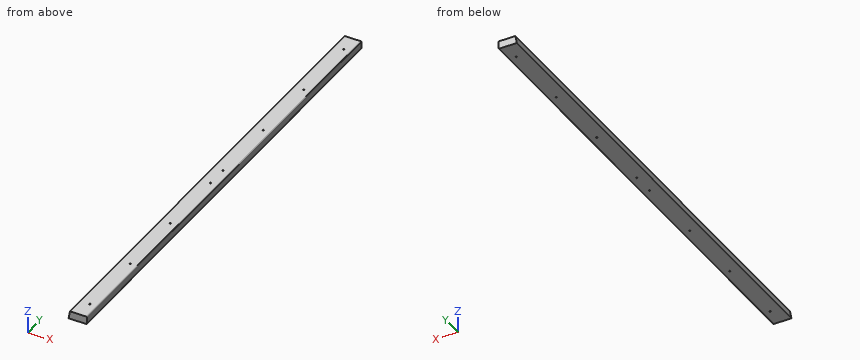
```python
from build123d import *

# Parameters (mm, degrees)
BOSS_EXTRUDE1_DEPTH         = 2362.2
F_1_4_0_25_DIAMETER_HOLE1_D = 6.35
FILLET2_R                   = 3.175


with BuildPart() as part:
    # Sketch1 → Boss-Extrude1 (new body)
    with BuildSketch(Plane(origin=(0, 0, 0), x_dir=(1, 0, 0), z_dir=(0, 1, 0))):
        Polygon((-44.45, 19.05), (-37.731942035, -19.05), (44.45, -19.05), (44.45, 19.05), align=None)
    extrude(amount=BOSS_EXTRUDE1_DEPTH)

    # 1/4 (0.25) Diameter Hole1 (through all)
    with Locations(Plane(origin=(0, 0, 19.05), x_dir=(-1, 0, 0), z_dir=(0, 0, 1))):
        with Locations((-8.817444165, -88.9), (-8.817444165, -434.975), (-8.817444165, -781.05), (-8.817444165, -1127.125)):
            f_1_4_0_25_diameter_hole1 = Hole(F_1_4_0_25_DIAMETER_HOLE1_D / 2)

    # Fillet2
    fillet2_edges = [part.edges().sort_by_distance(p)[0] for p in [
        (44.45, 1181.1, 19.05),
        (44.45, 1181.1, -19.05),
    ]]
    fillet(fillet2_edges, radius=FILLET2_R)

    # Mirror1: 1/4 (0.25) Diameter Hole1 across plane
    add(f_1_4_0_25_diameter_hole1.mirror(Plane(origin=(0, 1181.1, 0), x_dir=(0, 0, 1), z_dir=(0, -1, 0))), mode=Mode.SUBTRACT)


solid = part.part
```
Part model, mm, in its own coordinate system. Coordinates: 2 decimals unless noted, no trailing zeros. Order: outer loops, then holes, each group sorted by start corner. A loop starts at its lowest first (then second) coordinate and runs counter-clockwise, first axis right, second up. Notation, with made-up numbers: (10, 20.25) - (61, 20.25) arc R17 cw to (61, 32.25) - close; hole circle Ø8 at (64, 88.5). An arc over 180 degrees is marked (long way). Return JSON: item names as keys, results as strings. Group by question number.
Item 1: Cut at A-A (y = 1508). List the corners of the cut face in (x, z) (3 decimals), plus the area to 3 significant figures.
Item 2: Cut at B-B (z = 1). State how many separate pieces and enclosed holes the cut face has, plus the area to 3 significant figures.
Item 3: Drill centre lines: probe 1 along X at (y, z) = (1581, 10); probe 2 along X at (y, z) = (88.9, 1); probe 3 along X at (y, z) = (196, -17). Where is each one in solid material? Low to high. Write a range as from..to.
Item 4: Pin check, flat tip, straight feed: pin 1 (4 mm diameter, centred on x = 8.82, y = 2273.3, fed in from -Z). Stop position of the tip, or through.
Check values:
{
 "1": {"outline": "(-44.45, -19.05) - (41.275, -19.05) arc R3.175 ccw to (44.45, -15.875) - (44.45, 15.875) arc R3.175 ccw to (41.275, 19.05) - (-37.732, 19.05) - close", "area": "3,250 mm2"},
 "2": {"separate pieces": "1", "enclosed holes": "8", "area": "201,000 mm2"},
 "3": {"probe 1": "x = -39.33..5.65, 11.99..44.45", "probe 2": "x = -40.91..5.64, 11.99..44.45", "probe 3": "x = -44.09..44.24"},
 "4": {"pin 1": "passes through"}
}
